Read the model definition and answer for the solid it produces. Units are mm, in the model's axes. A direction names the side the tool comes from. Give positions to 0.01 mm unless a question says otherwise; leave off trailing zeros. Write each loop counter-clockwise with the first axis right and the second up, starting at its lowest first coordinate (ties: lowest second). Pieces come first, ordered by that corner, then holes. Notation, with made-up numbers: M -36,-28 L -20,-28 A21 cw -20,10 Z; hole C 37.25,-11 d5. An arc over 180 degrees is marked long. Put each result on its own line as item: value.
Autodesk Inventor part; units mm, degrees
ref_plane "YZ Plane" through (0, 0, 0) normal (1, 0, 0) x (0, 1, 0)
ref_plane "XZ Plane" through (0, 0, 0) normal (0, 1, 0) x (-1, 0, 0)
ref_plane "XY Plane" through (0, 0, 0) normal (0, 0, 1) x (1, 0, 0)
sketch "Sketch1" plane through (0, 0, 0) normal (0, 0, 1) x (1, 0, 0)
  line L0 (5, 0) -> (5, 75)
  line L1 (5, 75) -> (0, 75) construction
  line L2 (5, 75) -> (55, 75) construction
  line L3 (40.3553, 110.3553) -> (30.3553, 110.3553)
  line L4 (30.3553, 110.3553) -> (0, 80)
  line L5 (0, 0) -> (0, 80) construction
  line L6 (5, 0) -> (2, 0)
  line L7 (2, 0) -> (3.5, 2.5981)
  line L8 (3.5, 2.5981) -> (0, 2.5981)
  line L9 (-5, 0) -> (-5, 75)
  line L10 (-5, 75) -> (-40.3553, 110.3553)
  line L11 (-40.3553, 110.3553) -> (-30.3553, 110.3553)
  line L12 (-30.3553, 110.3553) -> (0, 80)
  line L13 (-5, 0) -> (-2, 0)
  line L14 (-2, 0) -> (-3.5, 2.5981)
  line L15 (-3.5, 2.5981) -> (0, 2.5981)
  line L16 (10, 80) -> (10, 85)
  line L17 (10, 85) -> (15, 85)
  line L18 (5, 75) -> (10, 80)
  line L19 (15, 85) -> (40.3553, 110.3553)
  dimension "d0" = 5
  dimension "d1" = 75
  dimension "d2" = 50
  dimension "d5" = 10
  dimension "d6" = 3
  dimension "d7" = 3
  dimension "d8" = 60
  dimension "d9" = 5
  dimension "d15" = 45
  dimension "d16" = 5
  dimension "d17" = 5
extrude "Extrusion1" add sketch "Sketch1" along normal mid plane 3.175
properties part number "Liu_Inital_Y"
(1) Given pin 1 Ø1.6 at (x, z) = (0.5, -0.5) entering from -Y; pin 2 Ø1.5 at (y, z) = (58.5, -0.5) entering from -X; pin 3 Ø10 at (x, y) = (14.5, 44) entering from -Z; pin 4 Ø1 at (y, z) = (19.5, 0.5) entering from +X, each flat-ended and moving along its own axis, determine where each tip first touches the part or whether it passes through.
Result:
pin 1: stops at y = 2.6
pin 2: stops at x = -5
pin 3: passes through
pin 4: stops at x = 5
(2) Section C-C on x = 13.5 is taken. Determine the outline of the cut face in (y, z), and give its area (3 significant figures).
Result:
outline: M 85,-1.59 L 93.5,-1.59 L 93.5,1.59 L 85,1.59 Z
area: 27.0 mm²
(3) Section D-D on y = 38.5 is taken. Determine the outline of the cut face in (x, z), and give its area (4 significant figures).
Result:
outline: M -5,-1.59 L 5,-1.59 L 5,1.59 L -5,1.59 Z
area: 31.75 mm²
(4) Straight lines are drawn through the part: line 1 along X through (y, z) = (18.5, -1); line 2 along X through (y, z) = (97.5, -0.05); line 3 along X through (y, z) = (95.5, -0.8). For each, find the intervals that lie inside material, in ascending order. Write a range as from..to.
Result:
line 1: x = -5..5
line 2: x = -27.5..-17.5, 17.5..27.5
line 3: x = -25.5..-15.5, 15.5..25.5
(5) Section A-A on y = 102.5 is taken. Determine the outline of the cut face in (x, z), and give its area (3 significant figures).
Result:
outline: M -32.5,-1.59 L -22.5,-1.59 L -22.5,1.59 L -32.5,1.59 Z; M 22.5,-1.59 L 32.5,-1.59 L 32.5,1.59 L 22.5,1.59 Z
area: 63.5 mm²
(6) Which of the six approach directions +Z, -Z, +X, -X, +Y, -Y give full straight-line access (tool end or side, diameter ignored) to faces 5 (the face through (-5, 37, 0)), 6 (the face through (35, 110.355, 0)), 7 (the face through (12, 85, 0)), 8 (the face through (15, 95, 0))?
Result:
face 5: +Z, -Z, -X, -Y
face 6: +Z, -Z, +X, -X, +Y
face 7: +Z, -Z, +X, -Y
face 8: +Z, -Z, +Y
(7) For a pull along X with two mould halves and no side action, classify faces 1 (the face through (2.74, 1.28, -0.02)), 2 (the face through (10, 82, 0)), 3 (the face through (-4, 0, 0)), 4 (the face through (-2.74, 1.28, -0.02)) as +X half, -X half, draft (parallel to the pull), parting line (faces both ways), or undercut.
Result:
face 1: undercut
face 2: +X half
face 3: draft
face 4: undercut
(8) Section B-B on z = 0.95 is taken. Determine the outline of the cut face in (x, y).
Result:
outline: M -40.36,110.36 L -5,75 L -5,0 L -2,0 L -3.5,2.6 L 3.5,2.6 L 2,0 L 5,0 L 5,75 L 10,80 L 10,85 L 15,85 L 40.36,110.36 L 30.36,110.36 L 0,80 L -30.36,110.36 Z
